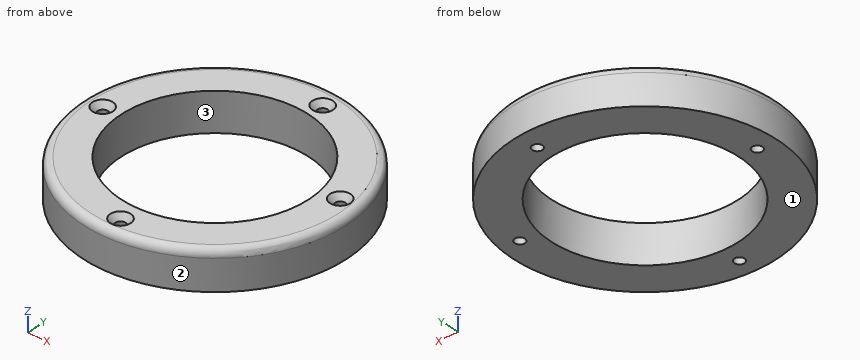
from build123d import *

# Parameters (mm, degrees)
F0_R           = 86.927765
F0_R_2         = 61.88106
F1_DEPTH       = 25.4
F3_D           = 6.7564
F3_CSINK_D     = 13.4874
F3_CSINK_ANGLE = 82
F4_R           = 5.08


with BuildPart() as f1:
    # F0 (on Top) → F1 (new body)
    with BuildSketch(Plane.XY):
        Circle(F0_R)
        Circle(F0_R_2, mode=Mode.SUBTRACT)
    extrude(amount=F1_DEPTH)

    # F3 (through all)
    with Locations(Plane.XY.offset(25.4)):
        with Locations((-73.593527, 0), (0, -74.825756), (73.592886, 10.307162), (11.192732, 71.860947)):
            CounterSinkHole(F3_D / 2, F3_CSINK_D / 2, counter_sink_angle=F3_CSINK_ANGLE)

    # F4
    f4_edges = [f1.edges().sort_by_distance(p)[0] for p in [
        (-86.927765, 0, 25.4),
    ]]
    fillet(f4_edges, radius=F4_R)


solid = f1.part
Part model, mm, in its own coordinate system. Face numbers are marked on the shaded views. Give positions to 0.01 mm unless a question says otherwise; leave off trailing zeros. Write each loop counter-clockwise with the first axis right and the second up, starting at its lowest first coordinate (ties: lowest second). Pieces come first, ordered by that corner, then holes.
1) Cut at C-C on z = 6. Write the cut outline in (x, y), then the cut area to 3 significant figures.
Resolved:
outline: circle Ø173.86 at (0, 0); hole circle Ø6.76 at (-73.59, 0); hole circle Ø123.76 at (0, 0); hole circle Ø6.76 at (0, -74.83); hole circle Ø6.76 at (11.19, 71.86); hole circle Ø6.76 at (73.59, 10.31)
area: 11,600 mm2
2) Cut at A-A on y = 0. Write the cut outline in (x, z).
Resolved:
outline: (-86.93, 0) - (-76.97, 0) - (-76.97, 21.53) - (-80.34, 25.4) - (-81.85, 25.4) arc R5.08 ccw to (-86.93, 20.32) - close; (-70.22, 0) - (-61.88, 0) - (-61.88, 25.4) - (-66.85, 25.4) - (-70.22, 21.53) - close; (61.88, 0) - (86.93, 0) - (86.93, 20.32) arc R5.08 ccw to (81.85, 25.4) - (61.88, 25.4) - close
3) Cut at B-B on x = 0. Write the cut outline in (y, z).
Resolved:
outline: (-86.93, 0) - (-78.2, 0) - (-78.2, 21.53) - (-81.57, 25.4) - (-81.85, 25.4) arc R5.08 ccw to (-86.93, 20.32) - close; (-71.45, 0) - (-61.88, 0) - (-61.88, 25.4) - (-68.08, 25.4) - (-71.45, 21.53) - close; (61.88, 0) - (86.93, 0) - (86.93, 20.32) arc R5.08 ccw to (81.85, 25.4) - (61.88, 25.4) - close
4) Two-plate mould, pull along X, no slides. Class the marked faces 1, 2 and 3: released by +X, released by -X, zero draft, split by the parting line, or undercut.
Resolved:
face 1: zero draft
face 2: split by the parting line
face 3: undercut
5) Probe L1, parallel to Y at x = 0, z = 4.5; L2, parallel to Y at x = 13.5, z = 15.5; L3, parallel to Y at x = 20.5, z = 13. List the from-to ranges inside material, lowest first.
Resolved:
L1: y = -86.93 to -78.2, -71.45 to -61.88, 61.88 to 86.93
L2: y = -85.87 to -60.39, 60.39 to 69.39, 74.33 to 85.87
L3: y = -84.48 to -58.39, 58.39 to 84.48
6) Pin check, flat tips, straight feed: pin 1 (4 mm diameter, centred on x = -58, z = 5.5, fed in from +Y); pin 2 (11 mm diameter, centred on x = 0, y = -74.83, fed in from +Z); pin 3 (9 mm diameter, centred on x = -73.59, y = 0, fed in from +Z); pin 4 (5 mm diameter, centred on x = -62.5, y = -53.5, fed in from -Z). Stop position of each tip, or through.
Resolved:
pin 1: stops at y = 66.49
pin 2: stops at z = 23.97
pin 3: stops at z = 22.82
pin 4: stops at z = 0
